from build123d import *

# Parameters (mm, degrees)
SKETCH1_W           = 20
SKETCH1_H           = 20
BOSS_EXTRUDE1_DEPTH = 14
CUT_EXTRUDE1_DEPTH  = 12


with BuildPart() as part:
    # Sketch1 → Boss-Extrude1 (new body)
    with BuildSketch(Plane.XY):
        Rectangle(SKETCH1_W, SKETCH1_H)
    extrude(amount=BOSS_EXTRUDE1_DEPTH)

    # Sketch2 → Cut-Extrude1 (cut)
    with BuildSketch(Plane(origin=(0, 0, 0), x_dir=(-1, 0, 0), z_dir=(0, 0, -1))):
        Polygon((3, 8), (-8, 8), (-8, -8), (-5, -8), (-5, -10), (10, -10), (10, 10), (5, 10), (5, 3), (3, 3), align=None)
    extrude(amount=-CUT_EXTRUDE1_DEPTH, mode=Mode.SUBTRACT)


solid = part.part
Design review of the part built by this model. Coordinates are the model's own, in mm. A direction names the side the tool comes from. Coordinates: 2 decimals unless noted, no trailing zeros. Order: outer loops, then holes, each group sorted by start corner. A loop starts at its lowest first (then second) coordinate and runs counter-clockwise, first axis right, second up. Notation, with made-up numbers: (-34.5, 81) -> (-3.5, 81) arc R17 ccw to (-3.5, 113) -> close; hole circle Ø4 at (64, 53). An arc over 180 degrees is marked (long way). One line per item, written item: value.
1) Clearance check with flat-ended pins moving along their axes: P1, Ø0.6, axis at x = -4.5, z = 8, coming from the -Y side; P2, Ø3.5, axis at y = -1, z = 3.5, coming from the -X side; P3, Ø1, axis at y = -9, z = 8.5, coming from the -X side. State where each tip first meets the part, or that it passes through.
Output values:
P1: stops at y = 3
P2: stops at x = 8
P3: stops at x = 5
2) Machinability: for faces 4 (the face through (7, -8, 6)), 5 (the face through (5, -9, 6)), 6 (the face through (-3, 5, 6)), 7 (the face through (-5, 7, 6)), which of the approach directions +Z, -Z, +X, -X, +Y, -Y give a long, thin tool a straight path to every point of the face, cutting with its end or side? Answer none if there is none.
Output values:
face 4: -Z, -X
face 5: -Z, -X, -Y
face 6: -Z, -Y
face 7: -Z, -X, +Y, -Y
3) Draft analysis for pull direction Y (two halves, no side actions). For faces 1 (the face through (8, 0, 6)), 2 (the face through (2, 10, 7)), 3 (the face through (0, 0, 14)), state which applies: +Y half, -Y half, draft (parallel to the pull), parting line (faces both ways), or undercut.
Output values:
face 1: undercut
face 2: +Y half
face 3: draft
4) We need section B-B, the plane x = 6. Give the boundary of the cut face in (y, z), then the cut area to 3 significant figures.
Output values:
outline: (-10, 0) -> (-8, 0) -> (-8, 12) -> (8, 12) -> (8, 0) -> (10, 0) -> (10, 14) -> (-10, 14) -> close
area: 88.0 mm2
5) To check wall thickness, follow probe 1 along Y at (x, z) = (7.5, 4.75); probe 2 along X at (y, z) = (3.5, 8.5); probe 3 along X at (y, z) = (1.25, 2.25). State the ranges of each line that lie inside material, in increasing order. Write a range as [from, to].
Output values:
probe 1: y = [-10, -8], [8, 10]
probe 2: x = [-5, -3], [8, 10]
probe 3: x = [8, 10]
6) We need section A-A, the plane y = 3.5. Give the boundary of the cut face in (x, z), then the cut area to 3 significant figures.
Output values:
outline: (-10, 12) -> (-5, 12) -> (-5, 0) -> (-3, 0) -> (-3, 12) -> (8, 12) -> (8, 0) -> (10, 0) -> (10, 14) -> (-10, 14) -> close
area: 88.0 mm2
7) We need section C-C, the plane z = 3.25. Give the boundary of the cut face in (x, y).
Output values:
outline: (-5, 3) -> (-3, 3) -> (-3, 8) -> (8, 8) -> (8, -8) -> (5, -8) -> (5, -10) -> (10, -10) -> (10, 10) -> (-5, 10) -> close
8) We need section D-D, the plane y = -1. Give the boundary of the cut face in (x, z), then the cut area to 3 significant figures.
Output values:
outline: (-10, 12) -> (8, 12) -> (8, 0) -> (10, 0) -> (10, 14) -> (-10, 14) -> close
area: 64.0 mm2
